Source: CAD feature listing. Evaluate the final solid. Frame: model axes, mm. Face numbers are marked on the shaded views. A direction names the side the tool comes from. Give positions to 0.01 mm unless a question says otherwise; leave off trailing zeros. Loops run counter-clockwise (first coordinate to the right, second up) from the corner with the lowest first, then second, coordinate; pieces in that order, holes last. Notation, with made-up numbers: M -26,44.25 L 3,44.25 A21 cw 3,49.25 Z; hole C 19.25,89 d3. An arc over 180 degrees is marked long. Write item = value, one per line.
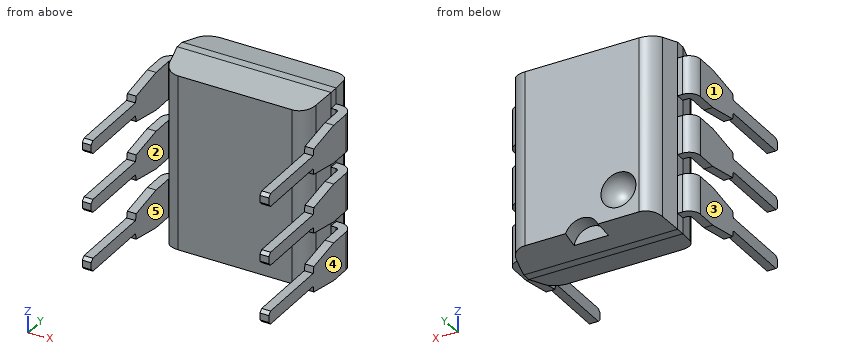
from build123d import *

# Parameters (mm, degrees)
BASE_EXTRUDE_DEPTH      = 6.58
BASE_EXTRUDE_DEPTH_BACK = 1.5
SKETCH1_W               = 6.6
SKETCH1_H               = 3.18
SKETCH2_OUTSIDE_W       = 10.782
SKETCH2_OUTSIDE_H       = 7.362
CUT_EXTRUDE1_DEPTH      = 12.593731065
SKETCH3_OUTSIDE_W       = 12.262
SKETCH3_OUTSIDE_H       = 7.362
CUT_EXTRUDE2_DEPTH      = 11.268032918
SKETCH5_W               = 1.63
SKETCH5_H               = 0.38
BOSS_EXTRUDE3_DEPTH     = 0.7
SKETCH6_W               = 0.38
SKETCH6_H               = 1.63
BOSS_EXTRUDE4_DEPTH     = 2.53
SKETCH4_W               = 0.38
SKETCH4_H               = 0.56
BOSS_EXTRUDE5_DEPTH     = 3.28
CUT_EXTRUDE5_DEPTH      = 0.38
FILLET1_R               = 0.49
FILLET2_R               = 0.11
FILLET1_OF_MIRROR1_R    = 0.49
FILLET2_OF_MIRROR1_R    = 0.11
LPATTERN1_START         = 0.3
LPATTERN1_OUTLINE_W     = 0.38
LPATTERN1_OUTLINE_H     = 1.63
LPATTERN1_DEPTH         = 7.02
LPATTERN1_START_2       = 1.725
LPATTERN1_2_DEPTH       = 1.63
LPATTERN1_START_3       = 4.265
LPATTERN1_3_DEPTH       = 1.63
LPATTERN1_START_4       = -0.19
LPATTERN1_4_DEPTH       = 0.38
LPATTERN1_START_5       = 7.43
LPATTERN1_5_DEPTH       = 0.38
SKETCH9_R               = 0.75
CUT_EXTRUDE6_DEPTH      = 0.7


with BuildPart() as part:
    # Sketch1 → Base-Extrude (new, two sides: drawn at the far end of the back side and taken through both)
    with BuildSketch(Plane.XY.offset(-BASE_EXTRUDE_DEPTH_BACK)):
        with Locations((3.81, 2.72)):
            Rectangle(SKETCH1_W, SKETCH1_H)
    extrude(amount=BASE_EXTRUDE_DEPTH + BASE_EXTRUDE_DEPTH_BACK)

    # Sketch2 outside → Cut-Extrude1 (cut, through all)
    with BuildSketch(Plane.XY.offset(6.58)):
        with Locations((3.81, 2.72)):
            Rectangle(SKETCH2_OUTSIDE_W, SKETCH2_OUTSIDE_H)
        with BuildLine():
            Line((0.51, 2.91), (0.679431307, 3.748623606))
            ThreePointArc((0.679431307, 3.748623606), (0.922305346, 4.151773257), (1.365567952, 4.31))
            Line((1.365567952, 4.31), (6.254432048, 4.31))
            ThreePointArc((6.254432048, 4.31), (6.697694654, 4.151773257), (6.940568693, 3.748623606))
            Line((6.940568693, 3.748623606), (7.11, 2.91))
            Line((7.11, 2.91), (7.11, 2.53))
            Line((7.11, 2.53), (6.940568693, 1.691376394))
            ThreePointArc((6.940568693, 1.691376394), (6.697694654, 1.288226743), (6.254432048, 1.13))
            Line((6.254432048, 1.13), (1.365567952, 1.13))
            ThreePointArc((1.365567952, 1.13), (0.922305346, 1.288226743), (0.679431307, 1.691376394))
            Line((0.679431307, 1.691376394), (0.51, 2.53))
            Line((0.51, 2.53), (0.51, 2.91))
        make_face(mode=Mode.SUBTRACT)
    extrude(amount=-CUT_EXTRUDE1_DEPTH, mode=Mode.SUBTRACT)

    # Sketch3 outside → Cut-Extrude2 (cut, through all)
    with BuildSketch(Plane(origin=(7.11, 0, 0), x_dir=(0, 0, -1), z_dir=(1, 0, 0))):
        with Locations((-2.54, 2.72)):
            Rectangle(SKETCH3_OUTSIDE_W, SKETCH3_OUTSIDE_H)
        Polygon((1.5, 2.91), (1.134316679, 4.72), (-6.214316679, 4.72), (-6.58, 2.91), (-6.58, 2.53), (-6.214316679, 0.72), (1.134316679, 0.72), (1.5, 2.53), align=None, mode=Mode.SUBTRACT)
    extrude(amount=-CUT_EXTRUDE2_DEPTH, mode=Mode.SUBTRACT)

    # Sketch5 → Boss-Extrude3 (add)
    with BuildSketch(Plane.ZY.offset(-0.51)):
        with Locations((0, 2.72)):
            Rectangle(SKETCH5_W, SKETCH5_H)
    boss_extrude3 = extrude(amount=BOSS_EXTRUDE3_DEPTH)

    # Sketch8 → Cut-Revolve1 (revolve, cut)
    with BuildSketch(Plane.XY):
        with BuildLine():
            Line((2.237663013, 3.56), (2.237663013, 4.31))
            Line((2.237663013, 4.31), (2.987663013, 4.31))
            ThreePointArc((2.987663013, 4.31), (2.767993099, 3.779669914), (2.237663013, 3.56))
        make_face()
    revolve(axis=Axis((2.237663013, 4.928970116, 0), (0, -1, 0)), mode=Mode.SUBTRACT)

    # Sketch6 → Boss-Extrude4 (add)
    with BuildSketch(Plane.XZ.offset(-2.53)):
        Rectangle(SKETCH6_W, SKETCH6_H)
    boss_extrude4 = extrude(amount=BOSS_EXTRUDE4_DEPTH)

    # Sketch4 → Boss-Extrude5 (add)
    with BuildSketch(Plane(origin=(0, 0, 0), x_dir=(1, 0, 0), z_dir=(0, 1, 0))):
        Rectangle(SKETCH4_W, SKETCH4_H)
    boss_extrude5 = extrude(amount=-BOSS_EXTRUDE5_DEPTH)

    # Sketch7 → Cut-Extrude5 (cut)
    with BuildSketch(Plane.ZY.offset(0.19)):
        Polygon((0.815, 1.52), (0.55, 0.05), (0.28, 0), (0.28, -3.15), (0.15, -3.28), (-0.15, -3.28), (-0.28, -3.15), (-0.28, 0), (-0.55, 0.05), (-0.815, 1.52), (-0.815, -3.78), (0.815, -3.78), align=None)
    cut_extrude5 = extrude(amount=-CUT_EXTRUDE5_DEPTH, mode=Mode.SUBTRACT)

    # Fillet1
    fillet1_edges = [part.edges().sort_by_distance(p)[0] for p in [
        (-0.19, 2.91, 0),
    ]]
    fillet(fillet1_edges, radius=FILLET1_R)

    # Fillet2
    fillet2_edges = [part.edges().sort_by_distance(p)[0] for p in [
        (0.19, 2.53, 0),
    ]]
    fillet(fillet2_edges, radius=FILLET2_R)

    # Mirror1: Boss-Extrude3, Boss-Extrude4, Boss-Extrude5, Cut-Extrude5 across plane
    add(boss_extrude3.mirror(Plane.ZY.offset(-3.81)))
    add(boss_extrude4.mirror(Plane.ZY.offset(-3.81)))
    add(boss_extrude5.mirror(Plane.ZY.offset(-3.81)))
    add(cut_extrude5.mirror(Plane.ZY.offset(-3.81)), mode=Mode.SUBTRACT)

    # Fillet1 of Mirror1
    fillet1_of_mirror1_edges = [part.edges().sort_by_distance(p)[0] for p in [
        (7.81, 2.91, 0),
    ]]
    fillet(fillet1_of_mirror1_edges, radius=FILLET1_OF_MIRROR1_R)

    # Fillet2 of Mirror1
    fillet2_of_mirror1_edges = [part.edges().sort_by_distance(p)[0] for p in [
        (7.43, 2.53, 0),
    ]]
    fillet(fillet2_of_mirror1_edges, radius=FILLET2_OF_MIRROR1_R)

    # LPattern1: read off the stored shape, not the designer's step
    # LPattern1 outline → LPattern1 (add)
    with BuildSketch(Plane.YZ.offset(LPATTERN1_START)):
        with Locations((2.72, 5.08)):
            Rectangle(LPATTERN1_OUTLINE_W, LPATTERN1_OUTLINE_H)
        with Locations((2.72, 2.54)):
            Rectangle(LPATTERN1_OUTLINE_W, LPATTERN1_OUTLINE_H)
    extrude(amount=LPATTERN1_DEPTH)

    # LPattern1 2 outline → LPattern1 2 (add)
    with BuildSketch(Plane.XY.offset(LPATTERN1_START_2)):
        with BuildLine():
            Line((7.43, -3.28), (7.81, -3.28))
            Line((7.81, -3.28), (7.81, 2.42))
            ThreePointArc((7.81, 2.42), (7.666482323, 2.766482323), (7.32, 2.91))
            Line((7.32, 2.91), (7.32, 2.53))
            ThreePointArc((7.32, 2.53), (7.397781746, 2.497781746), (7.43, 2.42))
            Line((7.43, 2.42), (7.43, -3.28))
        make_face()
        with BuildLine():
            Line((-0.19, 2.42), (-0.19, -3.28))
            Line((-0.19, -3.28), (0.19, -3.28))
            Line((0.19, -3.28), (0.19, 2.42))
            ThreePointArc((0.19, 2.42), (0.222218254, 2.497781746), (0.3, 2.53))
            Line((0.3, 2.53), (0.3, 2.91))
            ThreePointArc((0.3, 2.91), (-0.046482323, 2.766482323), (-0.19, 2.42))
        make_face()
    extrude(amount=LPATTERN1_2_DEPTH)

    # LPattern1 3 outline → LPattern1 3 (add)
    with BuildSketch(Plane.XY.offset(LPATTERN1_START_3)):
        with BuildLine():
            Line((7.43, -3.28), (7.81, -3.28))
            Line((7.81, -3.28), (7.81, 2.42))
            ThreePointArc((7.81, 2.42), (7.666482323, 2.766482323), (7.32, 2.91))
            Line((7.32, 2.91), (7.32, 2.53))
            ThreePointArc((7.32, 2.53), (7.397781746, 2.497781746), (7.43, 2.42))
            Line((7.43, 2.42), (7.43, -3.28))
        make_face()
        with BuildLine():
            Line((-0.19, 2.42), (-0.19, -3.28))
            Line((-0.19, -3.28), (0.19, -3.28))
            Line((0.19, -3.28), (0.19, 2.42))
            ThreePointArc((0.19, 2.42), (0.222218254, 2.497781746), (0.3, 2.53))
            Line((0.3, 2.53), (0.3, 2.91))
            ThreePointArc((0.3, 2.91), (-0.046482323, 2.766482323), (-0.19, 2.42))
        make_face()
    extrude(amount=LPATTERN1_3_DEPTH)

    # LPattern1 4 outline → LPattern1 4 (cut)
    with BuildSketch(Plane.YZ.offset(LPATTERN1_START_4)):
        Polygon((-3.28, 5.23), (-3.15, 5.36), (0, 5.36), (0.05, 5.63), (1.52, 5.895), (-3.28, 5.895), align=None)
        Polygon((-3.15, 4.8), (-3.28, 4.93), (-3.28, 4.265), (1.52, 4.265), (0.05, 4.53), (0, 4.8), align=None)
        Polygon((-3.28, 2.69), (-3.15, 2.82), (0, 2.82), (0.05, 3.09), (1.52, 3.355), (-3.28, 3.355), align=None)
        Polygon((-3.15, 2.26), (-3.28, 2.39), (-3.28, 1.725), (1.52, 1.725), (0.05, 1.99), (0, 2.26), align=None)
    extrude(amount=LPATTERN1_4_DEPTH, mode=Mode.SUBTRACT)

    # LPattern1 5 outline → LPattern1 5 (cut)
    with BuildSketch(Plane.YZ.offset(LPATTERN1_START_5)):
        Polygon((-3.28, 5.23), (-3.15, 5.36), (0, 5.36), (0.05, 5.63), (1.52, 5.895), (-3.28, 5.895), align=None)
        Polygon((-3.15, 4.8), (-3.28, 4.93), (-3.28, 4.265), (1.52, 4.265), (0.05, 4.53), (0, 4.8), align=None)
        Polygon((-3.28, 2.69), (-3.15, 2.82), (0, 2.82), (0.05, 3.09), (1.52, 3.355), (-3.28, 3.355), align=None)
        Polygon((-3.15, 2.26), (-3.28, 2.39), (-3.28, 1.725), (1.52, 1.725), (0.05, 1.99), (0, 2.26), align=None)
    extrude(amount=LPATTERN1_5_DEPTH, mode=Mode.SUBTRACT)

    # Sketch9 → Cut-Extrude6 (cut)
    with BuildSketch(Plane(origin=(0, 4.31, 0), x_dir=(-1, 0, 0), z_dir=(0, 1, 0))):
        with Locations((-3.81, -1.5)):
            Circle(SKETCH9_R)
    extrude(amount=-CUT_EXTRUDE6_DEPTH, mode=Mode.SUBTRACT)


solid = part.part
1. Pull-direction query (X, two-part tool) for the marked faces 3, 4 and 5; classes: +X half, -X half, draft (parallel to the pull), parting line (faces both ways), or undercut.
Derived:
face_3 = -X half
face_4 = +X half
face_5 = undercut
2. Material intervals for probe 1 along X at (y, z) = (-1.75, 0); probe 2 along X at (y, z) = (2, 0.75); probe 3 along X at (y, z) = (2.25, 5), sorted ascending. Write a range as from..to.
Derived:
probe_1 = -0.19..0.19, 7.43..7.81
probe_2 = -0.19..0.19, 0.62..7, 7.43..7.81
probe_3 = -0.19..0.19, 0.57..7.05, 7.43..7.81
3. Cut plane A-A, the plane y = 0.5. Return the cut outline in (x, z).
Derived:
outline = M -0.19,-0.63 L 0.19,-0.63 L 0.19,0.63 L -0.19,0.63 Z; M -0.19,1.91 L 0.19,1.91 L 0.19,3.17 L -0.19,3.17 Z; M -0.19,4.45 L 0.19,4.45 L 0.19,5.71 L -0.19,5.71 Z; M 7.43,-0.63 L 7.81,-0.63 L 7.81,0.63 L 7.43,0.63 Z; M 7.43,1.91 L 7.81,1.91 L 7.81,3.17 L 7.43,3.17 Z; M 7.43,4.45 L 7.81,4.45 L 7.81,5.71 L 7.43,5.71 Z
4. Cut plane C-C, the plane z = 1.5. Return the cut outline in (x, y), then the cut area to 3 significant figures.
Derived:
outline = M 0.51,2.53 L 0.68,1.69 A0.7 ccw 1.37,1.13 L 6.25,1.13 A0.7 ccw 6.94,1.69 L 7.11,2.53 L 7.11,2.91 L 6.94,3.75 A0.7 ccw 6.25,4.31 L 1.37,4.31 A0.7 ccw 0.68,3.75 L 0.51,2.91 Z
area = 19.9 mm²
5. First-contact query: pin 1 Ø0.6 at (x, y) = (0, 2.5) entering from +Z (3 decimals); pin 2 Ø1.5 at (x, z) = (0.5, 1) entering from +Y. Flat tips, straight axial feed; report the tip coordinate or a pass-through.
Derived:
pin_1 = 5.895
pin_2 = 4.3
6. Reachability of the marked faces 1 and 2 from +Z, -Z, +X, -X, +Y, -Y: full face, straight path, thin tool, end or side. Return the list, or none.
Derived:
face_1 = +Z, -Z, -X, +Y, -Y
face_2 = +Z, -Z, -Y
7. Cut plane D-D, the plane y = -1.75. Return the cut outline in (x, z), then the cut area to 3 significant figures.
Derived:
outline = M -0.19,-0.28 L 0.19,-0.28 L 0.19,0.28 L -0.19,0.28 Z; M -0.19,2.26 L 0.19,2.26 L 0.19,2.82 L -0.19,2.82 Z; M -0.19,4.8 L 0.19,4.8 L 0.19,5.36 L -0.19,5.36 Z; M 7.43,-0.28 L 7.81,-0.28 L 7.81,0.28 L 7.43,0.28 Z; M 7.43,2.26 L 7.81,2.26 L 7.81,2.82 L 7.43,2.82 Z; M 7.43,4.8 L 7.81,4.8 L 7.81,5.36 L 7.43,5.36 Z
area = 1.28 mm²
8. Cut plane B-B, the plane x = 5.75. Return the cut outline in (y, z), then the cut area to 3 significant figures.
Derived:
outline = M 1.13,-1.22 L 2.53,-1.5 L 2.91,-1.5 L 4.31,-1.22 L 4.31,6.3 L 2.91,6.58 L 2.53,6.58 L 1.13,6.3 Z
area = 24.9 mm²
